Here's how the part is built. I have some questions about the finished solid (model axes, mm). Face numbers are marked on the shaded views. A direction names the side the tool comes from. Give positions to 0.01 mm unless a question says otherwise; leave off trailing zeros. Loops run counter-clockwise (first coordinate to the right, second up) from the corner with the lowest first, then second, coordinate; pieces in that order, holes last. Notation, with made-up numbers: (86, -11) - (116, -11) arc R21 cw to (116, 6) - close; hole circle Ø10 at (21.25, 51.25). An arc over 180 degrees is marked (long way). Put each result on its own line as item: value. Start each with the question number.
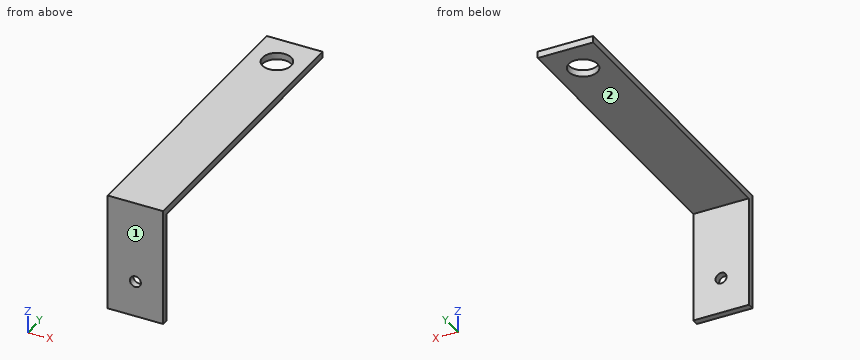
from build123d import *

# Parameters (mm, degrees)
CROQUIS1_W              = 50
CROQUIS1_H              = 100
SALIENTE_EXTRUIR1_DEPTH = 6
CROQUIS2_W              = 50
CROQUIS2_H              = 6
SALIENTE_EXTRUIR2_DEPTH = 270
CROQUIS3_R              = 13
CORTAR_EXTRUIR1_DEPTH   = 107
SKETCH1_R               = 5
CUT_EXTRUDE1_DEPTH      = 10


with BuildPart() as part:
    # Croquis1 → Saliente-Extruir1 (new body)
    with BuildSketch(Plane(origin=(0, 0, 0), x_dir=(1, 0, 0), z_dir=(0, 1, 0))):
        Rectangle(CROQUIS1_W, CROQUIS1_H)
    extrude(amount=SALIENTE_EXTRUIR1_DEPTH)

    # Croquis2 → Saliente-Extruir2 (add)
    with BuildSketch(Plane.XZ):
        with Locations((0, 53)):
            Rectangle(CROQUIS2_W, CROQUIS2_H)
    extrude(amount=-SALIENTE_EXTRUIR2_DEPTH)

    # Croquis3 → Cortar-Extruir1 (cut, through all)
    with BuildSketch(Plane.XY.offset(56)):
        with Locations((0, 240)):
            Circle(CROQUIS3_R)
    extrude(amount=-CORTAR_EXTRUIR1_DEPTH, mode=Mode.SUBTRACT)

    # Sketch1 → Cut-Extrude1 (cut)
    with BuildSketch(Plane(origin=(0, 6, 0), x_dir=(1, 0, 0), z_dir=(0, 1, 0))):
        with Locations((0, 17.616363636)):
            Circle(SKETCH1_R)
    extrude(amount=-CUT_EXTRUDE1_DEPTH, mode=Mode.SUBTRACT)


solid = part.part
1) Suppose I cut it at D-D on y = 47.5. Please give me the cut outline in (x, z).
2) I need wall thicknesses on line 1 (Z direction, x = 0, y = 1.7); line 2 (Z direction, x = -0.5, y = 198); line 3 (Y direction, x = -11, z = 29). Which ranges of each line are inside material? Lowest first, please.
3) Suppose I cut it at A-A on y = 240. Please give me the cut outline in (x, z), plus the area to 3 significant figures.
4) I'm going to push flat-ended pins straight in: P1, Ø1, axis at x = -7.5, y = 188.5, coming from the -Z side; P2, Ø15, axis at x = -1.5, z = 12.5, coming from the +Y side. Where does each tip first touch, or does it pass through?
5) Suppose I cut it at C-C on x = -22. Please give me the cut outline in (y, z), plus the area to 3 significant figures.
6) Suppose I cut it at B-B on x = 0. Please give me the cut outline in (y, z), plus the area to 3 significant figures.
7) Which directions (+Z, -Z, +X, -X, +Y, -Y) give clear straight access to the entire face, cutting with the end or side of a thin tool? Please do the marked faces 1 and 2.
Ans:
1. outline: (-25, 50) - (25, 50) - (25, 56) - (-25, 56) - close
2. line 1: z = -50 to -22.62, -12.62 to 56
2. line 2: z = 50 to 56
2. line 3: y = 0 to 6
3. outline: (-25, 50) - (-13, 50) - (-13, 56) - (-25, 56) - close; (13, 50) - (25, 50) - (25, 56) - (13, 56) - close
3. area: 144 mm²
4. P1: stops at z = 50
4. P2: stops at y = 6
5. outline: (0, -50) - (6, -50) - (6, 50) - (270, 50) - (270, 56) - (0, 56) - close
5. area: 2,220 mm²
6. outline: (0, -50) - (6, -50) - (6, -22.62) - (0, -22.62) - close; (0, -12.62) - (6, -12.62) - (6, 50) - (227, 50) - (227, 56) - (0, 56) - close; (253, 50) - (270, 50) - (270, 56) - (253, 56) - close
6. area: 2,000 mm²
7. face 1: +Z, -Z, +X, -X, -Y
7. face 2: -Z, +X, -X, +Y
